from build123d import *

# Parameters (mm, degrees)
BOSS_EXTRUDE1_DEPTH      = 1.27
BOSS_EXTRUDE1_DEPTH_BACK = 1.27
SKETCH1_R                = 1.27
BOSS_EXTRUDE2_START      = 2.54
SKETCH3_R                = 1.27
BOSS_EXTRUDE2_DEPTH      = 2.54
SKETCH4_W                = 11.43
SKETCH4_H                = 2.54
CUT_EXTRUDE2_DEPTH       = 15.199031657


with BuildPart() as part:
    # Sketch1 → Boss-Extrude1 (new, two sides: drawn at the far end of the back side and taken through both)
    with BuildSketch(Plane.XY.offset(-BOSS_EXTRUDE1_DEPTH_BACK)):
        with BuildLine():
            Line((-10.16, 2.54), (10.16, 2.54))
            ThreePointArc((10.16, 2.54), (12.7, 0), (10.16, -2.54))
            Line((10.16, -2.54), (-10.16, -2.54))
            ThreePointArc((-10.16, -2.54), (-12.7, 0), (-10.16, 2.54))
        make_face()
        with Locations((-10.16, 0)):
            Circle(SKETCH1_R, mode=Mode.SUBTRACT)
        with Locations((10.16, 0)):
            Circle(SKETCH1_R, mode=Mode.SUBTRACT)
    extrude(amount=BOSS_EXTRUDE1_DEPTH + BOSS_EXTRUDE1_DEPTH_BACK)

    # Sketch3 → Boss-Extrude2 (add)
    with BuildSketch(Plane(origin=(0, 0, -1.27), x_dir=(-1, 0, 0), z_dir=(0, 0, -1)).offset(BOSS_EXTRUDE2_START)):
        with BuildLine():
            Line((2.54, -2.54), (2.54, 2.54))
            Line((2.54, 2.54), (-10.16, 2.54))
            ThreePointArc((-10.16, 2.54), (-12.7, 0), (-10.16, -2.54))
            Line((-10.16, -2.54), (2.54, -2.54))
        make_face()
        with Locations(Location((-10.16, 0, 0), (0, 0, 180))):
            Circle(SKETCH3_R, mode=Mode.SUBTRACT)
    extrude(amount=-BOSS_EXTRUDE2_DEPTH)

    # Sketch4 → Cut-Extrude2 (cut, through all)
    with BuildSketch(Plane(origin=(0, 2.54, 0), x_dir=(1, 0, 0), z_dir=(0, 1, 0))):
        with Locations((6.985, 0)):
            Rectangle(SKETCH4_W, SKETCH4_H)
    extrude(amount=-CUT_EXTRUDE2_DEPTH, mode=Mode.SUBTRACT)


solid = part.part
The listing builds one solid part. Answer for the finished solid, in the listing's coordinates (mm). A direction names the side the tool comes from. Give positions to 0.01 mm unless a question says otherwise; leave off trailing zeros. Order: outer loops, then holes, each group sorted by start corner. A loop starts at its lowest first (then second) coordinate and runs counter-clockwise, first axis right, second up. Notation, with made-up numbers: (43.25, 71.25) - (47.25, 71.25) arc R27 cw to (47.25, 90.25) - close; hole circle Ø4 at (-29.75, 65). An arc over 180 degrees is marked (long way). One line per item, written item: value. Start each with the question number.
1) A cutting plane is placed at A-A on z = -0.95. Give the vertices of the cut face in (x, y), then the cut area to 3 significant figures.
2) A cutting plane is placed at D-D on y = -1.9. Give the vertices of the cut face in (x, z), then the cut area to 3 significant figures.
3) Given pin 1 Ø3 at (x, z) = (6.5, -1) entering from -Y; pin 2 Ø1.3 at (y, z) = (1, -0.5) entering from +X; pin 3 Ø1.5 at (x, y) = (6.5, -0.5) entering from +Z; pin 4 Ø0.8 at (y, z) = (-1, -2.5) entering from -X, each flat-ended and moving along its own axis, determine where each tip first touches the part or whether it passes through.
4) Find the intervals of material crossed by L1, parallel to Y at x = 10.16, z = -2.2; L2, parallel to Z at x = -3, y = -2.1; L3, parallel to Z at x = 3, y = 1.55, in increasing order.
5) A cutting plane is placed at B-B on y = -0.75. Give the vertices of the cut face in (x, z), then the cut area to 3 significant figures.
6) A cutting plane is placed at C-C on z = -2.7. Give the vertices of the cut face in (x, y), then the cut area to 3 significant figures.
7) A tool of negligible diameter and unlimited length cuts with its end or side. For faces 4 (the face through (1.27, 0, 0)), 5 (the face through (-8, 0, -1.27)), 6 (the face through (-6, 0, 1.27)), from which of +Z, -Z, +X, -X, +Y, -Y can it reach the whole face along a straight path? Write none if from no direction.
8) The mould has two halves that part along Y. Classify faces 1 (the face through (12.7, 0.1, -2.6)), 2 (the face through (5, 0, -3.81)), 3 (the face through (-8.99, -0.49, -0.02)): released by +Y, released by -Y, zero draft, split by the parting line, or undercut.
Answer sheet:
1. outline: (-10.16, -2.54) - (1.27, -2.54) - (1.27, 2.54) - (-10.16, 2.54) arc R2.54 ccw to start; hole circle Ø2.54 at (-10.16, 0)
1. area: 63.1 mm2
2. outline: (-11.85, -1.27) - (-2.54, -1.27) - (-2.54, -3.81) - (11.85, -3.81) - (11.85, -1.27) - (1.27, -1.27) - (1.27, 1.27) - (-11.85, 1.27) - close
2. area: 69.9 mm2
3. pin 1: stops at y = -2.54
3. pin 2: stops at x = 1.27
3. pin 3: stops at z = -1.27
3. pin 4: stops at x = -2.54
4. L1: y = -2.54 to -1.27, 1.27 to 2.54
4. L2: z = -1.27 to 1.27
4. L3: z = -3.81 to -1.27
5. outline: (-12.59, -1.27) - (-11.18, -1.27) - (-11.18, 1.27) - (-12.59, 1.27) - close; (-9.14, -1.27) - (-2.54, -1.27) - (-2.54, -3.81) - (9.14, -3.81) - (9.14, -1.27) - (1.27, -1.27) - (1.27, 1.27) - (-9.14, 1.27) - close; (11.18, -3.81) - (12.59, -3.81) - (12.59, -1.27) - (11.18, -1.27) - close
5. area: 63.2 mm2
6. outline: (-2.54, -2.54) - (10.16, -2.54) arc R2.54 ccw to (10.16, 2.54) - (-2.54, 2.54) - close; hole circle Ø2.54 at (10.16, 0)
6. area: 69.6 mm2
7. face 4: +Z, +X, +Y, -Y
7. face 5: -Z, -X, +Y, -Y
7. face 6: +Z, +X, -X, +Y, -Y
8. face 1: split by the parting line
8. face 2: zero draft
8. face 3: undercut
